Design review of the part built by this model. Coordinates are the model's own, in mm. A direction names the side the tool comes from. Coordinates: 2 decimals unless noted, no trailing zeros. Order: outer loops, then holes, each group sorted by start corner. A loop starts at its lowest first (then second) coordinate and runs counter-clockwise, first axis right, second up. Notation, with made-up numbers: (-1, 65.25) -> (18, 65.25) arc R25 cw to (18, 89.25) -> close; hole circle Ø9 at (-40, 42). An arc over 180 degrees is marked (long way). Write item = value, one per line.
```python
from build123d import *

# Parameters (mm, degrees)
F0_W     = 630
F0_H     = 50
F1_DEPTH = 2200
F2_T     = -2.5
F4_DEPTH = 30


with BuildPart() as f1:
    # F0 (on Front) → F1 (new body)
    with BuildSketch(Plane.XZ):
        with Locations((315, 25)):
            Rectangle(F0_W, F0_H)
    extrude(amount=F1_DEPTH)

    # F2
    f2_openings = [f1.faces().sort_by_distance(p)[0] for p in [
        (315, -1100, 50),
    ]]
    offset(amount=F2_T, openings=f2_openings)

    # F3 (on face) → F4 (cut)
    with BuildSketch(Plane.XZ.offset(2.5)):
        with BuildLine():
            ThreePointArc((52.5, 2.5), (61.338835, 6.161165), (65, 15))
            ThreePointArc((65, 15), (43.661165, 23.838835), (52.5, 2.5))
        make_face()
    extrude(amount=-F4_DEPTH, mode=Mode.SUBTRACT)


solid = f1.part
```
(1) We need section C-C (x = 139). Write out the cut boundary in (y, z).
Report:
outline = (-2200, 0) -> (0, 0) -> (0, 50) -> (-2.5, 50) -> (-2.5, 2.5) -> (-2197.5, 2.5) -> (-2197.5, 50) -> (-2200, 50) -> close
(2) The part is to be moulded in two halves that separate along Y. For faces 1 (the flat face through (311, -2.5, 27)), 2 (the flat face through (311, -1085, 0)), 3 (the flat face through (311, 0, 25)), say which applies: released by +Y, released by -Y, zero draft, split by the parting line, or undercut.
Report:
face_1 = undercut
face_2 = zero draft
face_3 = released by +Y
(3) For L1, parallel to X at y = -215, z = 16; L2, parallel to X at y = -1, z = 15; L3, parallel to Y at x = 528, z = 4.5, list the stretches that pass through material, from the lowest coordinate up.
Report:
L1 = 0 to 2.5, 627.5 to 630
L2 = 0 to 40, 65 to 630
L3 = -2200 to -2197.5, -2.5 to 0
(4) Insertion check: pin 1 (2 mm diameter, centred on x = 419, y = -1378, fed in from +Z). The pin has a flat end and moves straight along its axis. Give the tip position at first contact, or say it passes through.
Report:
pin_1 = 2.5
(5) We need section A-A (z = 42). Write out the cut boundary in (x, y), and give its area (3 significant figures).
Report:
outline = (0, -2200) -> (630, -2200) -> (630, 0) -> (0, 0) -> close; hole (2.5, -2197.5) -> (627.5, -2197.5) -> (627.5, -2.5) -> (2.5, -2.5) -> close
area = 14,100 mm²
(6) For faces 4 (the flat face through (311, -2200, 25)), 5 (the flat face through (311, -2197.5, 27)), list the 3-axis set-ups (+Z, -Z, +X, -X, +Y, -Y) from which the entire face can be reached by the end or side of a thin tool; tool diameter is ignored.
Report:
face_4 = +Z, -Z, +X, -X, -Y
face_5 = +Z
(7) We need section B-B (y = -790.5). Write out the cut boundary in (x, z), and give its area (3 significant figures).
Report:
outline = (0, 0) -> (630, 0) -> (630, 50) -> (627.5, 50) -> (627.5, 2.5) -> (2.5, 2.5) -> (2.5, 50) -> (0, 50) -> close
area = 1,810 mm²
